Could you check a few things on this model? Use its own coordinates, in mm. Face numbers are marked on the shaded views. A direction names the side the tool comes from. Round coordinates to 2 decimals unless told otherwise and drop trailing zeros. Loops run counter-clockwise (first coordinate to the right, second up) from the corner with the lowest first, then second, coordinate; pieces in that order, holes last.
from build123d import *

# Parameters (mm, degrees)
F0_R     = 4.446176
F1_DEPTH = 25.4


with BuildPart() as f1:
    # F0 (on Front) → F1 (new body)
    with BuildSketch(Plane.XZ):
        with BuildLine():
            ThreePointArc((27.262543, -8.093622), (28.143037, -4.089309), (28.438582, 0))
            ThreePointArc((28.438582, 0), (28.392606, 1.616437), (28.254827, 3.227648))
            ThreePointArc((28.254827, 3.227648), (-19.268549, 20.915926), (-5.529564, -27.895822))
            ThreePointArc((-5.529564, -27.895822), (0.429583, -28.435337), (6.369713, -27.716055))
            ThreePointArc((6.369713, -27.716055), (19.469004, -20.729468), (27.262543, -8.093622))
        make_face()
        with Locations((7.510159, 14.593512)):
            Circle(F0_R, mode=Mode.SUBTRACT)
        with BuildLine():
            ThreePointArc((28.254827, 3.227648), (28.392606, 1.616437), (28.438582, 0))
            ThreePointArc((28.438582, 0), (28.143037, -4.089309), (27.262543, -8.093622))
            Line((27.262543, -8.093622), (50.118111, -2.741527))
            Line((50.118111, -2.741527), (28.254827, 3.227648))
        make_face()
        with BuildLine():
            ThreePointArc((6.369713, -27.716055), (0.429583, -28.435337), (-5.529564, -27.895822))
            Line((-5.529564, -27.895822), (-5.529564, -53.295822))
            Line((-5.529564, -53.295822), (6.369713, -53.295822))
            Line((6.369713, -53.295822), (6.369713, -27.716055))
        make_face()
    extrude(amount=F1_DEPTH)


solid = f1.part
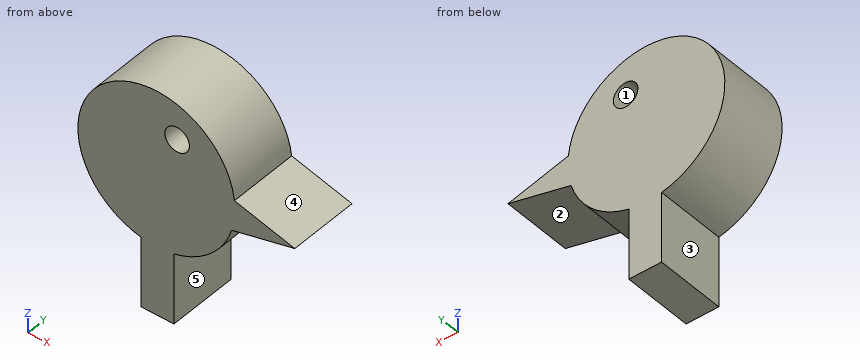
Item 1: If we section it at A-A, the plane y = -22: Please give me the cut outline in (x, z).
Results list:
outline: (-5.53, -53.3) - (6.37, -53.3) - (6.37, -27.72) arc R28.44 ccw to (27.26, -8.09) - (50.12, -2.74) - (28.25, 3.23) arc R28.44 ccw (long way) to (-5.53, -27.9) - close; hole circle Ø8.89 at (7.51, 14.59)
Item 2: If I drill on line 1 along Z through (x, y) = (-3, -12.25); line 2 along X through (y, z) = (-18.5, 17); line 3 along X through (y, z) = (-23.5, -38.5), over which ranges is the centre line in solid material (lowest first)?
Results list:
line 1: z = -53.3 to 28.28
line 2: x = -22.8 to 3.77, 11.25 to 22.8
line 3: x = -5.53 to 6.37
Item 3: If we section it at B-B, the plane z = -41: Please give me the cut outline in (x, y), then the cut area to 3 significant figures.
Results list:
outline: (-5.53, -25.4) - (6.37, -25.4) - (6.37, 0) - (-5.53, 0) - close
area: 302 mm2
Item 4: We'd pull the mould along X, two halves only. Please class the marked faces 1, 2 and 3: released by +X, released by -X, zero draft, split by the parting line, or undercut.
Results list:
face 1: undercut
face 2: released by +X
face 3: released by -X
Item 5: Will these pins go through, and if not, where does the flat tip stop? pin 1 (6 mm diameter, centred on y = -9, z = -28, fed in from -X); pin 2 (4 mm diameter, centred on x = -8, y = -3, fed in from -Z); pin 3 (2 mm diameter, centred on x = 21, y = -22.5, fed in from -Z).
Results list:
pin 1: stops at x = -13.56
pin 2: stops at z = -27.8
pin 3: stops at z = -20.22
Item 6: For the marked faces 4 and 5, which set-ups out of +Z, -Z, +X, -X, +Y, -Y let a thin tool reach every point of the face, with its end or its side?
Results list:
face 4: +Z, +X, +Y, -Y
face 5: -Z, +X, +Y, -Y
Item 7: If we section it at C-C, the plane x = 13: Please give me the cut outline in (y, z).
Results list:
outline: (-25.4, -25.29) - (0, -25.29) - (0, 25.29) - (-25.4, 25.29) - close
